```python
from build123d import *

# Parameters (mm, degrees)
BOSS_EXTRUDE1_DEPTH = 8
BOSS_EXTRUDE2_DEPTH = 10
SKETCH6_R           = 3
BOSS_EXTRUDE3_DEPTH = 1.5
SKETCH7_W           = 48.5
SKETCH7_H           = 4
CUT_EXTRUDE3_DEPTH  = 67.710194124
SKETCH8_W           = 13
SKETCH8_H           = 36.5
BOSS_EXTRUDE4_DEPTH = 10
SKETCH9_W           = 3
SKETCH9_H           = 28.7
CUT_EXTRUDE4_DEPTH  = 67.710194124
SKETCH10_R          = 1.6
CUT_EXTRUDE5_DEPTH  = 69.368486893
SKETCH11_R          = 3
CUT_EXTRUDE6_DEPTH  = 14
SKETCH12_R          = 1.45
CUT_EXTRUDE7_DEPTH  = 6
SKETCH13_W          = 13
SKETCH13_H          = 36.5
BOSS_EXTRUDE5_DEPTH = 5
SKETCH14_R          = 2
CUT_EXTRUDE8_DEPTH  = 5
FILLET1_R           = 1


with BuildPart() as part:
    # Sketch2 → Boss-Extrude1 (new body)
    with BuildSketch(Plane(origin=(0, 0, 0), x_dir=(1, 0, 0), z_dir=(0, 1, 0))):
        Polygon((-62, 6), (-45.5, 22.5), (45.5, 22.5), (62, 6), (62, -6), (45.5, -22.5), (-45.5, -22.5), (-62, -6), align=None)
    extrude(amount=BOSS_EXTRUDE1_DEPTH)

    # Sketch5 → Boss-Extrude2 (add)
    with BuildSketch(Plane(origin=(0, 8, 0), x_dir=(1, 0, 0), z_dir=(0, 1, 0))):
        Polygon((-62, 6), (-62, -6), (-45.5, -22.5), (45.5, -22.5), (62, -6), (62, 6), (45.5, 22.5), (-45.5, 22.5), align=None)
        with BuildLine():
            Line((-58, 4.343145751), (-58, -4.343145751))
            Line((-58, -4.343145751), (-46.671572875, -15.671572875))
            ThreePointArc((-46.671572875, -15.671572875), (-42.312412021, -14.80448187), (-39.843145751, -18.5))
            Line((-39.843145751, -18.5), (39.843145751, -18.5))
            ThreePointArc((39.843145751, -18.5), (42.312412021, -14.80448187), (46.671572875, -15.671572875))
            Line((46.671572875, -15.671572875), (58, -4.343145751))
            Line((58, -4.343145751), (58, 4.343145751))
            Line((58, 4.343145751), (46.671572875, 15.671572875))
            ThreePointArc((46.671572875, 15.671572875), (42.312412021, 14.80448187), (39.843145751, 18.5))
            Line((39.843145751, 18.5), (-39.843145751, 18.5))
            ThreePointArc((-39.843145751, 18.5), (-42.312412021, 14.80448187), (-46.671572875, 15.671572875))
            Line((-46.671572875, 15.671572875), (-58, 4.343145751))
        make_face(mode=Mode.SUBTRACT)
    extrude(amount=BOSS_EXTRUDE2_DEPTH)

    # Sketch6 → Boss-Extrude3 (add)
    with BuildSketch(Plane(origin=(0, 8, 0), x_dir=(1, 0, 0), z_dir=(0, 1, 0))):
        with Locations(Location((18, 14.35, 0), (0, 0, 90))):
            Circle(SKETCH6_R)
        with Locations(Location((-30.5, 14.35, 0), (0, 0, 90))):
            Circle(SKETCH6_R)
        with Locations(Location((-30.5, -14.35, 0), (0, 0, 90))):
            Circle(SKETCH6_R)
        with Locations(Location((18, -14.35, 0), (0, 0, 90))):
            Circle(SKETCH6_R)
    extrude(amount=BOSS_EXTRUDE3_DEPTH)

    # Sketch7 → Cut-Extrude3 (cut, through all)
    with BuildSketch(Plane(origin=(0, 8, 0), x_dir=(1, 0, 0), z_dir=(0, 1, 0))):
        with Locations((-6.25, 20.5)):
            Rectangle(SKETCH7_W, SKETCH7_H)
        with Locations((-6.25, -20.5)):
            Rectangle(SKETCH7_W, SKETCH7_H)
    extrude(amount=CUT_EXTRUDE3_DEPTH, mode=Mode.SUBTRACT)

    # Sketch8 → Boss-Extrude4 (add, through all)
    with BuildSketch(Plane(origin=(0, 8, 0), x_dir=(1, 0, 0), z_dir=(0, 1, 0))):
        with BuildLine():
            Line((23.843145751, 18.5), (23.843145751, -18.5))
            Line((23.843145751, -18.5), (39.843145751, -18.5))
            ThreePointArc((39.843145751, -18.5), (40.68086809, -16.050510257), (42.843145751, -14.627016654))
            Line((42.843145751, -14.627016654), (42.843145751, 14.627016654))
            ThreePointArc((42.843145751, 14.627016654), (40.68086809, 16.050510257), (39.843145751, 18.5))
            Line((39.843145751, 18.5), (23.843145751, 18.5))
        make_face()
        with Locations((33.343145751, 0)):
            Rectangle(SKETCH8_W, SKETCH8_H, mode=Mode.SUBTRACT)
    extrude(amount=BOSS_EXTRUDE4_DEPTH)

    # Sketch9 → Cut-Extrude4 (cut, through all)
    with BuildSketch(Plane(origin=(0, 8, 0), x_dir=(1, 0, 0), z_dir=(0, 1, 0))):
        with Locations((25.343145751, 0)):
            Rectangle(SKETCH9_W, SKETCH9_H)
    extrude(amount=CUT_EXTRUDE4_DEPTH, mode=Mode.SUBTRACT)

    # Sketch10 → Cut-Extrude5 (cut, through all)
    with BuildSketch(Plane(origin=(0, 18, 0), x_dir=(1, 0, 0), z_dir=(0, 1, 0))):
        with Locations(Location((-43.843145751, 18.5, 0), (0, 0, 270))):
            Circle(SKETCH10_R)
        with Locations(Location((43.843145751, 18.5, 0), (0, 0, 270))):
            Circle(SKETCH10_R)
        with Locations(Location((43.843145751, -18.5, 0), (0, 0, 270))):
            Circle(SKETCH10_R)
        with Locations(Location((-43.843145751, -18.5, 0), (0, 0, 270))):
            Circle(SKETCH10_R)
    extrude(amount=-CUT_EXTRUDE5_DEPTH, mode=Mode.SUBTRACT)

    # Sketch11 → Cut-Extrude6 (cut)
    with BuildSketch(Plane.XZ):
        with Locations(Location((-43.843145751, 18.5, 0), (0, 0, 270))):
            Circle(SKETCH11_R)
        with Locations(Location((43.843145751, 18.5, 0), (0, 0, 270))):
            Circle(SKETCH11_R)
        with Locations(Location((43.843145751, -18.5, 0), (0, 0, 270))):
            Circle(SKETCH11_R)
        with Locations(Location((-43.843145751, -18.5, 0), (0, 0, 270))):
            Circle(SKETCH11_R)
    extrude(amount=-CUT_EXTRUDE6_DEPTH, mode=Mode.SUBTRACT)

    # Sketch12 → Cut-Extrude7 (cut)
    with BuildSketch(Plane(origin=(0, 9.5, 0), x_dir=(1, 0, 0), z_dir=(0, 1, 0))):
        with Locations(Location((-30.5, 14.35, 0), (0, 0, 270))):
            Circle(SKETCH12_R)
        with Locations(Location((18, 14.35, 0), (0, 0, 270))):
            Circle(SKETCH12_R)
        with Locations(Location((18, -14.35, 0), (0, 0, 270))):
            Circle(SKETCH12_R)
        with Locations(Location((-30.5, -14.35, 0), (0, 0, 270))):
            Circle(SKETCH12_R)
    extrude(amount=-CUT_EXTRUDE7_DEPTH, mode=Mode.SUBTRACT)

    # Sketch13 → Boss-Extrude5 (add)
    with BuildSketch(Plane(origin=(0, 8, 0), x_dir=(1, 0, 0), z_dir=(0, 1, 0))):
        with Locations((33.343145751, 0)):
            Rectangle(SKETCH13_W, SKETCH13_H)
    extrude(amount=BOSS_EXTRUDE5_DEPTH)

    # Sketch14 → Cut-Extrude8 (cut)
    with BuildSketch(Plane.XZ):
        with Locations(Location((-13.435028843, 13.435028843, 0), (0, 0, 270))):
            Circle(SKETCH14_R)
        with Locations(Location((13.435028843, 13.435028843, 0), (0, 0, 270))):
            Circle(SKETCH14_R)
        with Locations(Location((13.435028843, -13.435028843, 0), (0, 0, 270))):
            Circle(SKETCH14_R)
        with Locations(Location((-13.435028843, -13.435028843, 0), (0, 0, 270))):
            Circle(SKETCH14_R)
    extrude(amount=-CUT_EXTRUDE8_DEPTH, mode=Mode.SUBTRACT)

    # Fillet1
    fillet1_edges = [part.edges().sort_by_distance(p)[0] for p in [
        (33.343145751, 13, -18.25),
        (33.343145751, 13, 18.25),
    ]]
    fillet(fillet1_edges, radius=FILLET1_R)


solid = part.part
```
The listing builds one solid part. Answer for the finished solid, in the listing's coordinates (mm). A direction names the side the tool comes from. Give positions to 0.01 mm unless a question says otherwise; leave off trailing zeros. Order: outer loops, then holes, each group sorted by start corner. A loop starts at its lowest first (then second) coordinate and runs counter-clockwise, first axis right, second up. Notation, with made-up numbers: M 48.25,-11 L 76.25,-11 A19 cw 76.25,0 Z; hole C 27,56 d10. An arc over 180 degrees is marked long. Put each result on its own line as item: value. Start each with the question number.
Item 1: Which of the six approach directions +Z, -Z, +X, -X, +Y, -Y give full straight-line access (tool end or side, diameter ignored) to faces 1 (the face through (42.28, 16.03, -18.85)), 2 (the face through (17.12, 6.54, -15.5)), 3 (the face through (13, 5, -13))?
Item 2: Find the intervals of material crossed by line 1 along X through (y, z) = (10.75, -4); line 2 along Z through (x, y) = (-13.5, 4.5); line 3 along Z through (x, y) = (44, 9.25), in increasing order.
Item 3: Flat-ended cylindrical pins translate along their axes: P1, Ø6.5, axis at x = 32.5, z = 4.5, coming from the +Y side; P2, Ø3.5, axis at x = -43.84, z = -18.5, coming from the -Y side; P3, Ø3, axis at x = 8.5, z = 1.5, coming from the +Y side; P4, Ø3, axis at x = 4, z = 3.5, coming from the -Y side. Find the tip coordinate at first contact, or state that the pin passes through.
Item 4: The part is cut by section A-A, the plane y = 2. State how many separate pieces and enclosed holes the cut face has, and give its area (3 significant figures).
Item 5: For a pull along X with two mould halves and no side action, classify faces 4 (the face through (-13, 5, 13)), 5 (the face through (-54, 9, 14)) as +X half, -X half, draft (parallel to the pull), parting line (faces both ways), or undercut.
Item 6: The part is cut by section C-C, the plane x = 6. Determine the outline of the cut face in (y, z).
Answer key:
1. face 1: +Y, -Y
1. face 2: +Y
1. face 3: -Y
2. line 1: x = -62 to -58, 26.84 to 42.84, 58 to 62
2. line 2: z = -22.5 to -15.43, -11.44 to 11.44, 15.43 to 22.5
2. line 3: z = -22.5 to -21.5, -15.5 to -14.5, 14.5 to 15.5, 21.5 to 22.5
3. P1: stops at y = 13
3. P2: stops at y = 14
3. P3: stops at y = 8
3. P4: stops at y = 0
4. separate pieces: 1
4. enclosed holes: 8
4. area: 4,870 mm²
5. face 4: undercut
5. face 5: -X half
6. outline: M 0,-22.5 L 8,-22.5 L 8,22.5 L 0,22.5 Z
